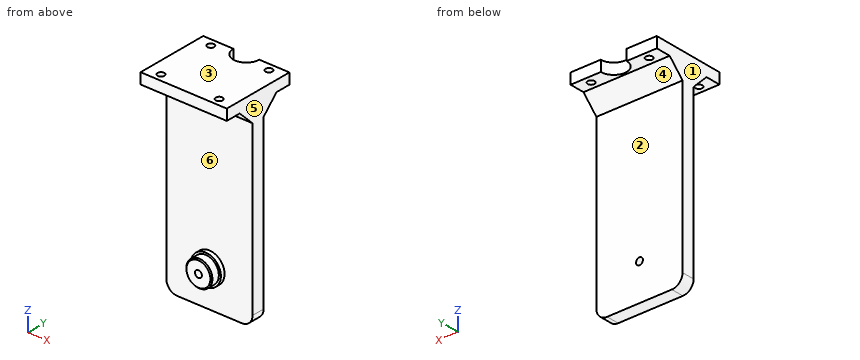
from build123d import *

# Parameters (mm, degrees)
SKETCH_1_W          = 40
SKETCH_1_H          = 95
EXTRUDE_1_DEPTH     = 6
SKETCH_2_W          = 40
SKETCH_2_H          = 5
EXTRUDE_2_DEPTH     = 14
SKETCH_3_R          = 6
CUT_EXTRUDE_1_DEPTH = 14
SKETCH_4_R          = 1.6
CUT_EXTRUDE_2_DEPTH = 14
CHAMFER_1_SIZE      = 7
FILLET_1_R          = 5
EXTRUDE_3_DEPTH     = 40
SKETCH_8_R          = 1.6
CUT_EXTRUDE_3_DEPTH = 40
SKETCH_5_R          = 7
EXTRUDE_4_DEPTH     = 2
SKETCH_9_R          = 6.05
EXTRUDE_5_DEPTH     = 4
CHAMFER_2_SIZE      = 0.5
SKETCH_10_R         = 1.6
CUT_EXTRUDE_4_DEPTH = 27


with BuildPart() as part:
    # Эскиз1 → Бобышка-Вытянуть1 (new body)
    with BuildSketch(Plane(origin=(0, 0, 0), x_dir=(1, 0, 0), z_dir=(0, 1, 0))):
        with Locations((0, 47.5)):
            Rectangle(SKETCH_1_W, SKETCH_1_H)
    extrude(amount=EXTRUDE_1_DEPTH)

    # Эскиз2 → Бобышка-Вытянуть2 (add)
    with BuildSketch(Plane(origin=(0, 6, 0), x_dir=(1, 0, 0), z_dir=(0, 1, 0))):
        with Locations((0, 2.5)):
            Rectangle(SKETCH_2_W, SKETCH_2_H)
    extrude(amount=EXTRUDE_2_DEPTH)

    # Эскиз3 → Вырез-Вытянуть1 (cut)
    with BuildSketch(Plane(origin=(0, 0, -5), x_dir=(-1, 0, 0), z_dir=(0, 0, -1))):
        with Locations((0, 20)):
            Circle(SKETCH_3_R)
    extrude(amount=-CUT_EXTRUDE_1_DEPTH, mode=Mode.SUBTRACT)

    # Эскиз4 → Вырез-Вытянуть2 (cut)
    with BuildSketch(Plane(origin=(0, 0, -5), x_dir=(-1, 0, 0), z_dir=(0, 0, -1))):
        with Locations((-13.5, 16.5)):
            Circle(SKETCH_4_R)
        with Locations((13.5, 16.5)):
            Circle(SKETCH_4_R)
    extrude(amount=-CUT_EXTRUDE_2_DEPTH, mode=Mode.SUBTRACT)

    # Фаска1
    chamfer_1_edges = [part.edges().sort_by_distance(p)[0] for p in [
        (0, 6, -5),
    ]]
    chamfer(chamfer_1_edges, length=CHAMFER_1_SIZE)

    # Скругление1
    fillet_1_edges = [part.edges().sort_by_distance(p)[0] for p in [
        (-20, 3, -95),
        (20, 3, -95),
    ]]
    fillet(fillet_1_edges, radius=FILLET_1_R)

    # Эскиз7 → Бобышка-Вытянуть3 (add)
    with BuildSketch(Plane.ZY.offset(20)):
        Polygon((0, -14), (-5, -14), (-5, -7), (-12, 0), (0, 0), align=None)
    extrude(amount=-EXTRUDE_3_DEPTH)

    # Эскиз8 → Вырез-Вытянуть3 (cut)
    with BuildSketch(Plane.XY):
        with Locations((13.5, 16.5)):
            Circle(SKETCH_8_R)
        with Locations((-13.5, 16.5)):
            Circle(SKETCH_8_R)
        with Locations((13.5, -10.5)):
            Circle(SKETCH_8_R)
        with Locations((-13.5, -10.5)):
            Circle(SKETCH_8_R)
    extrude(amount=-CUT_EXTRUDE_3_DEPTH, mode=Mode.SUBTRACT)

    # Эскиз5 → Бобышка-Вытянуть4 (add)
    with BuildSketch(Plane.XZ):
        with Locations((0, -78)):
            Circle(SKETCH_5_R)
    extrude(amount=EXTRUDE_4_DEPTH)

    # Эскиз9 → Бобышка-Вытянуть5 (add)
    with BuildSketch(Plane.XZ.offset(2)):
        with Locations((0, -78)):
            Circle(SKETCH_9_R)
    extrude(amount=EXTRUDE_5_DEPTH)

    # Фаска2
    chamfer_2_edges = [part.edges().sort_by_distance(p)[0] for p in [
        (-6.05, -6, -78),
    ]]
    chamfer(chamfer_2_edges, length=CHAMFER_2_SIZE)

    # Эскиз10 → Вырез-Вытянуть4 (cut, through all)
    with BuildSketch(Plane.XZ.offset(6)):
        with Locations((0, -78)):
            Circle(SKETCH_10_R)
    extrude(amount=-CUT_EXTRUDE_4_DEPTH, mode=Mode.SUBTRACT)


solid = part.part
Source: CAD feature listing. Evaluate the final solid. Frame: model axes, mm. Face numbers are marked on the shaded views. A direction names the side the tool comes from. Round coordinates to 2 decimals unless told otherwise and drop trailing zeros. Loops run counter-clockwise (first coordinate to the right, second up) from the corner with the lowest first, then second, coordinate; pieces in that order, holes last. Notation, with made-up numbers: M 24.25,84 L 82.25,84 A7 ccw 82.25,91 Z; hole C 26,72 d6. An arc over 180 degrees is marked long. Return JSON: item names as keys, results as strings. Group by question number.
1. Reachability of the marked faces 1 and 2 from +Z, -Z, +X, -X, +Y, -Y: full face, straight path, thin tool, end or side. Return the list, or none.
2. Section query A-A on x = 0. Output: boundary loops of the cut face in (y, z).
3. Pin query (flat end, axial travel): pin 1 (5 mm diameter, centred on x = 8, z = -52.5, fed in from -Y); pin 2 (5.5 mm diameter, centred on x = 6.5, y = -11.5, fed in from -Z); pin 3 (5 mm diameter, centred on x = 7.5, y = 10.5, fed in from -Z). Return the tip coordinate at first contact, or that it passes through.
4. Section query D-D on x = 13.5. Output: boundary loops of the cut face in (y, z).
5. Mould query, pull axis Z, two halves, no side actions, for the marked faces 3, 4, 5 and 6. Classes: released by +Z, released by -Z, zero draft, split by the parting line, or undercut.
6. Section query C-C on y = 16.5. Output: boundary loops of the cut face in (x, z), and give its area (3 significant figures).
7. Material intervals for line 1 along Y through (x, z) = (13.5, -3.5); line 2 along Z through (x, y) = (0, 0.5); line 3 along X through (y, z) = (-10, -3), sorted ascending. Write a range as from..to.
8. Section query B-B on z = -78. Output: boundary loops of the cut face in (x, y), and give its area (3 significant figures).
Checks:
{
 "1": {"face 1": "+Z, -Z, -X, +Y, -Y", "face 2": "-Z, +X, -X, +Y"},
 "2": {"outline": "M -14,-5 L -7,-5 L 0,-12 L 0,-71 L -2,-71 L -2,-71.95 L -5.5,-71.95 L -6,-72.45 L -6,-76.4 L 6,-76.4 L 6,-12 L 13,-5 L 14,-5 L 14,0 L -14,0 Z; M -6,-83.55 L -5.5,-84.05 L -2,-84.05 L -2,-85 L 0,-85 L 0,-95 L 6,-95 L 6,-79.6 L -6,-79.6 Z"},
 "3": {"pin 1": "stops at y = 0", "pin 2": "stops at z = -5", "pin 3": "stops at z = -10"},
 "4": {"outline": "M -14,-5 L -12.1,-5 L -12.1,0 L -14,0 Z; M -8.9,-5 L -7,-5 L 0,-12 L 0,-95 L 6,-95 L 6,-12 L 13,-5 L 14.9,-5 L 14.9,0 L -8.9,0 Z; M 18.1,-5 L 20,-5 L 20,0 L 18.1,0 Z"},
 "5": {"face 3": "released by +Z", "face 4": "released by -Z", "face 5": "zero draft", "face 6": "undercut"},
 "6": {"outline": "M -20,-5 L -15.1,-5 L -15.1,0 L -20,0 Z; M -11.9,-5 L -4.87,-5 L -4.87,0 L -11.9,0 Z; M 4.87,-5 L 11.9,-5 L 11.9,0 L 4.87,0 Z; M 15.1,-5 L 20,-5 L 20,0 L 15.1,0 Z", "area": "119 mm²"},
 "7": {"line 1": "y = -14..-12.1, -8.9..14.9, 18.1..20", "line 2": "z = -95..-79.6, -76.4..0", "line 3": "x = -20..-15.02, -11.98..11.98, 15.02..20"},
 "8": {"outline": "M -20,0 L -7,0 L -7,-2 L -6.05,-2 L -6.05,-5.5 L -5.55,-6 L -1.6,-6 L -1.6,6 L -20,6 Z; M 1.6,-6 L 5.55,-6 L 6.05,-5.5 L 6.05,-2 L 7,-2 L 7,0 L 20,0 L 20,6 L 1.6,6 Z", "area": "278 mm²"}
}
